from build123d import *

# Parameters (mm, degrees)
ESQUISSE1_R        = 2.15
BOSS_EXTRU_1_DEPTH = 297.5


with BuildPart() as part:
    # Esquisse1 → Boss.-Extru.1 (new, symmetric)
    with BuildSketch(Plane(origin=(0, 0, 0), x_dir=(-1, 0, 0), z_dir=(0, 0, -1))):
        with BuildLine():
            Line((-40, 6.7), (-40, 2))
            ThreePointArc((-40, 2), (-39.414213562, 0.585786438), (-38, 0))
            Line((-38, 0), (-33.3, 0))
            ThreePointArc((-33.3, 0), (-32.734314575, 0.234314575), (-32.5, 0.8))
            Line((-32.5, 0.8), (-32.5, 1.5))
            ThreePointArc((-32.5, 1.5), (-32.587867966, 1.712132034), (-32.8, 1.8))
            Line((-32.8, 1.8), (-34.918424061, 1.8))
            ThreePointArc((-34.918424061, 1.8), (-35.686700051, 2.313345604), (-35.506437047, 3.219588924))
            Line((-35.506437047, 3.219588924), (-33.254705627, 5.471320344))
            ThreePointArc((-33.254705627, 5.471320344), (-32.281435581, 6.121638598), (-31.133385284, 6.35))
            Line((-31.133385284, 6.35), (-28.866614716, 6.35))
            ThreePointArc((-28.866614716, 6.35), (-27.718564419, 6.121638598), (-26.745294373, 5.471320344))
            Line((-26.745294373, 5.471320344), (-24.493562953, 3.219588924))
            ThreePointArc((-24.493562953, 3.219588924), (-24.313299949, 2.313345604), (-25.081575939, 1.8))
            Line((-25.081575939, 1.8), (-27.2, 1.8))
            ThreePointArc((-27.2, 1.8), (-27.412132034, 1.712132034), (-27.5, 1.5))
            Line((-27.5, 1.5), (-27.5, 0.8))
            ThreePointArc((-27.5, 0.8), (-27.265685425, 0.234314575), (-26.7, 0))
            Line((-26.7, 0), (-13.3, 0))
            ThreePointArc((-13.3, 0), (-12.734314575, 0.234314575), (-12.5, 0.8))
            Line((-12.5, 0.8), (-12.5, 1.5))
            ThreePointArc((-12.5, 1.5), (-12.587867966, 1.712132034), (-12.8, 1.8))
            Line((-12.8, 1.8), (-14.918424061, 1.8))
            ThreePointArc((-14.918424061, 1.8), (-15.686700051, 2.313345604), (-15.506437047, 3.219588924))
            Line((-15.506437047, 3.219588924), (-13.254705627, 5.471320344))
            ThreePointArc((-13.254705627, 5.471320344), (-12.281435581, 6.121638598), (-11.133385284, 6.35))
            Line((-11.133385284, 6.35), (-8.866614716, 6.35))
            ThreePointArc((-8.866614716, 6.35), (-7.718564419, 6.121638598), (-6.745294373, 5.471320344))
            Line((-6.745294373, 5.471320344), (-4.493562953, 3.219588924))
            ThreePointArc((-4.493562953, 3.219588924), (-4.313299949, 2.313345604), (-5.081575939, 1.8))
            Line((-5.081575939, 1.8), (-7.2, 1.8))
            ThreePointArc((-7.2, 1.8), (-7.412132034, 1.712132034), (-7.5, 1.5))
            Line((-7.5, 1.5), (-7.5, 0.8))
            ThreePointArc((-7.5, 0.8), (-7.265685425, 0.234314575), (-6.7, 0))
            Line((-6.7, 0), (-2, 0))
            ThreePointArc((-2, 0), (-0.585786438, 0.585786438), (0, 2))
            Line((0, 2), (0, 6.7))
            ThreePointArc((0, 6.7), (-0.234314575, 7.265685425), (-0.8, 7.5))
            Line((-0.8, 7.5), (-1.5, 7.5))
            ThreePointArc((-1.5, 7.5), (-1.712132034, 7.412132034), (-1.8, 7.2))
            Line((-1.8, 7.2), (-1.8, 5.081575939))
            ThreePointArc((-1.8, 5.081575939), (-2.313345604, 4.313299949), (-3.219588924, 4.493562953))
            Line((-3.219588924, 4.493562953), (-5.471320344, 6.745294373))
            ThreePointArc((-5.471320344, 6.745294373), (-6.121638598, 7.718564419), (-6.35, 8.866614716))
            Line((-6.35, 8.866614716), (-6.35, 11.133385284))
            ThreePointArc((-6.35, 11.133385284), (-6.121638598, 12.281435581), (-5.471320344, 13.254705627))
            Line((-5.471320344, 13.254705627), (-3.219588924, 15.506437047))
            ThreePointArc((-3.219588924, 15.506437047), (-2.313345604, 15.686700051), (-1.8, 14.918424061))
            Line((-1.8, 14.918424061), (-1.8, 12.8))
            ThreePointArc((-1.8, 12.8), (-1.712132034, 12.587867966), (-1.5, 12.5))
            Line((-1.5, 12.5), (-0.8, 12.5))
            ThreePointArc((-0.8, 12.5), (-0.234314575, 12.734314575), (0, 13.3))
            Line((0, 13.3), (0, 18))
            ThreePointArc((0, 18), (-0.585786438, 19.414213562), (-2, 20))
            Line((-2, 20), (-6.7, 20))
            ThreePointArc((-6.7, 20), (-7.265685425, 19.765685425), (-7.5, 19.2))
            Line((-7.5, 19.2), (-7.5, 18.5))
            ThreePointArc((-7.5, 18.5), (-7.412132034, 18.287867966), (-7.2, 18.2))
            Line((-7.2, 18.2), (-5.081575939, 18.2))
            ThreePointArc((-5.081575939, 18.2), (-4.313299949, 17.686654396), (-4.493562953, 16.780411076))
            Line((-4.493562953, 16.780411076), (-6.745294373, 14.528679656))
            ThreePointArc((-6.745294373, 14.528679656), (-7.718564419, 13.878361402), (-8.866614716, 13.65))
            Line((-8.866614716, 13.65), (-11.133385284, 13.65))
            ThreePointArc((-11.133385284, 13.65), (-12.281435581, 13.878361402), (-13.254705627, 14.528679656))
            Line((-13.254705627, 14.528679656), (-15.506437047, 16.780411076))
            ThreePointArc((-15.506437047, 16.780411076), (-15.686700051, 17.686654396), (-14.918424061, 18.2))
            Line((-14.918424061, 18.2), (-12.8, 18.2))
            ThreePointArc((-12.8, 18.2), (-12.587867966, 18.287867966), (-12.5, 18.5))
            Line((-12.5, 18.5), (-12.5, 19.2))
            ThreePointArc((-12.5, 19.2), (-12.734314575, 19.765685425), (-13.3, 20))
            Line((-13.3, 20), (-26.7, 20))
            ThreePointArc((-26.7, 20), (-27.265685425, 19.765685425), (-27.5, 19.2))
            Line((-27.5, 19.2), (-27.5, 18.5))
            ThreePointArc((-27.5, 18.5), (-27.412132034, 18.287867966), (-27.2, 18.2))
            Line((-27.2, 18.2), (-25.081575939, 18.2))
            ThreePointArc((-25.081575939, 18.2), (-24.313299949, 17.686654396), (-24.493562953, 16.780411076))
            Line((-24.493562953, 16.780411076), (-26.745294373, 14.528679656))
            ThreePointArc((-26.745294373, 14.528679656), (-27.718564419, 13.878361402), (-28.866614716, 13.65))
            Line((-28.866614716, 13.65), (-31.133385284, 13.65))
            ThreePointArc((-31.133385284, 13.65), (-32.281435581, 13.878361402), (-33.254705627, 14.528679656))
            Line((-33.254705627, 14.528679656), (-35.506437047, 16.780411076))
            ThreePointArc((-35.506437047, 16.780411076), (-35.686700051, 17.686654396), (-34.918424061, 18.2))
            Line((-34.918424061, 18.2), (-32.8, 18.2))
            ThreePointArc((-32.8, 18.2), (-32.587867966, 18.287867966), (-32.5, 18.5))
            Line((-32.5, 18.5), (-32.5, 19.2))
            ThreePointArc((-32.5, 19.2), (-32.734314575, 19.765685425), (-33.3, 20))
            Line((-33.3, 20), (-38, 20))
            ThreePointArc((-38, 20), (-39.414213562, 19.414213562), (-40, 18))
            Line((-40, 18), (-40, 13.3))
            ThreePointArc((-40, 13.3), (-39.765685425, 12.734314575), (-39.2, 12.5))
            Line((-39.2, 12.5), (-38.5, 12.5))
            ThreePointArc((-38.5, 12.5), (-38.287867966, 12.587867966), (-38.2, 12.8))
            Line((-38.2, 12.8), (-38.2, 14.918424061))
            ThreePointArc((-38.2, 14.918424061), (-37.686654396, 15.686700051), (-36.780411076, 15.506437047))
            Line((-36.780411076, 15.506437047), (-34.528679656, 13.254705627))
            ThreePointArc((-34.528679656, 13.254705627), (-33.878361402, 12.281435581), (-33.65, 11.133385284))
            Line((-33.65, 11.133385284), (-33.65, 8.866614716))
            ThreePointArc((-33.65, 8.866614716), (-33.878361402, 7.718564419), (-34.528679656, 6.745294373))
            Line((-34.528679656, 6.745294373), (-36.780411076, 4.493562953))
            ThreePointArc((-36.780411076, 4.493562953), (-37.686654396, 4.313299949), (-38.2, 5.081575939))
            Line((-38.2, 5.081575939), (-38.2, 7.2))
            ThreePointArc((-38.2, 7.2), (-38.287867966, 7.412132034), (-38.5, 7.5))
            Line((-38.5, 7.5), (-39.2, 7.5))
            ThreePointArc((-39.2, 7.5), (-39.765685425, 7.265685425), (-40, 6.7))
        make_face()
        with Locations(Location((-10, 10, 0), (0, 0, 180))):
            Circle(ESQUISSE1_R, mode=Mode.SUBTRACT)
        with Locations(Location((-30, 10, 0), (0, 0, 180))):
            Circle(ESQUISSE1_R, mode=Mode.SUBTRACT)
        with BuildLine():
            Line((-18.585786174, 17.312993861), (-14.528681072, 13.255889759))
            ThreePointArc((-14.528681072, 13.255889759), (-13.878362627, 12.282619622), (-13.650001154, 11.134569154))
            Line((-13.650001154, 11.134569154), (-13.650001154, 8.865431094))
            ThreePointArc((-13.650001154, 8.865431094), (-13.878362476, 7.717381202), (-14.5286805, 6.7441115))
            Line((-14.5286805, 6.7441115), (-18.585786, 2.687006))
            ThreePointArc((-18.585786, 2.687006), (-19.999999562, 2.101219562), (-21.414213125, 2.687006))
            Line((-21.414213125, 2.687006), (-25.471320125, 6.744113))
            ThreePointArc((-25.471320125, 6.744113), (-26.121638379, 7.717383046), (-26.349999781, 8.865433344))
            Line((-26.349999781, 8.865433344), (-26.349999781, 11.134567344))
            ThreePointArc((-26.349999781, 11.134567344), (-26.121638308, 12.282617811), (-25.471319863, 13.255887949))
            Line((-25.471319863, 13.255887949), (-21.41421295, 17.312993861))
            ThreePointArc((-21.41421295, 17.312993861), (-19.999999562, 17.898780125), (-18.585786174, 17.312993861))
        make_face(mode=Mode.SUBTRACT)
    extrude(amount=BOSS_EXTRU_1_DEPTH, both=True)


solid = part.part
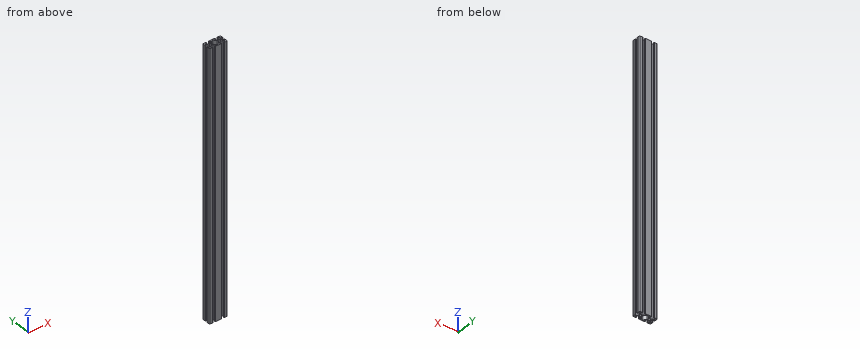
Input: part model. Units: mm. Frame: model coordinates. Round coordinates to 2 decimals unless told otherwise and drop trailing zeros. Answer as a JSON object with one key per item and string values. Group by question number.
1) Ray query, L1, parallel to X at y = 10, z = -28.5; L2, parallel to X at y = 14.5, z = -151; L3, parallel to X at y = 16, z = -202.5. Return the intervals inside material, ascending.
2) Section query A-A on z = 97. State how many separate pieces and enclosed holes the cut face has, plus the area to 3 significant figures.
3) Pin query (flat end, axial travel): pin 1 (0.8 mm diameter, centred on y = 1, z = 98, fed in from -X); pin 2 (1 mm diameter, centred on x = 10, z = 158, fed in from -Y); pin 3 (12 mm diameter, centred on y = 6.5, z = -114.5, fed in from -X); pin 4 (2.5 mm diameter, centred on x = 29.5, z = -134, fed in from +Y). Return the tip coordinate at first contact, or that it passes through.
Reply:
{
 "1": {"L1": "x = 6.35 to 7.85, 12.15 to 13.65, 26.35 to 27.85, 32.15 to 33.65", "L2": "x = 0 to 1.8, 4.23 to 6.77, 13.23 to 15.77, 24.23 to 26.77, 33.23 to 35.77, 38.2 to 40", "L3": "x = 0 to 5.27, 14.73 to 17.27, 22.73 to 25.27, 34.73 to 40"},
 "2": {"separate pieces": "1", "enclosed holes": "3", "area": "332 mm2"},
 "3": {"pin 1": "stops at x = 0.09", "pin 2": "stops at y = 6.35", "pin 3": "stops at x = 0", "pin 4": "stops at y = 13.71"}
}
